Work out the finished part from the listing and answer in its coordinate system (mm). A direction names the side the tool comes from. Coordinates: 2 decimals unless noted, no trailing zeros. Loops run counter-clockwise (first coordinate to the right, second up) from the corner with the lowest first, then second, coordinate; pieces in that order, holes last. Notation, with made-up numbers: (-4, 14) -> (33, 14) arc R16 cw to (33, 37) -> close; hole circle Ø3 at (17, 70.25). An arc over 180 degrees is marked (long way). Use a Markdown table: item, result.
from build123d import *

# Parameters (mm, degrees)
SKETCH1_R                    = 9.45
BOSS_EXTRUDE1_DEPTH          = 7
SKETCH2_R                    = 8.95
BOSS_EXTRUDE2_DEPTH          = 2
SKETCH3_R                    = 9.45
BOSS_EXTRUDE3_DEPTH          = 7
SKETCH4_R                    = 4
CUT_EXTRUDE1_DEPTH           = 21.847182064
M2_5X0_45_TAPPED_HOLE1_D     = 2.1
M2_5X0_45_TAPPED_HOLE1_DEPTH = 7
M2_5X0_45_TAPPED_HOLE1_TIP   = 0.63090365
M2_5X0_45_TAPPED_HOLE2_D     = 2.1
M2_5X0_45_TAPPED_HOLE2_DEPTH = 7
M2_5X0_45_TAPPED_HOLE2_TIP   = 0.63090365


with BuildPart() as part:
    # Sketch1 → Boss-Extrude1 (new body)
    with BuildSketch(Plane.XY):
        Circle(SKETCH1_R)
    extrude(amount=BOSS_EXTRUDE1_DEPTH)

    # Sketch2 → Boss-Extrude2 (add)
    with BuildSketch(Plane.XY.offset(7)):
        Circle(SKETCH2_R)
    extrude(amount=BOSS_EXTRUDE2_DEPTH)

    # Sketch3 → Boss-Extrude3 (add)
    with BuildSketch(Plane.XY.offset(9)):
        Circle(SKETCH3_R)
    extrude(amount=BOSS_EXTRUDE3_DEPTH)

    # Sketch4 → Cut-Extrude1 (cut, through all)
    with BuildSketch(Plane.XY.offset(16)):
        Circle(SKETCH4_R)
    extrude(amount=-CUT_EXTRUDE1_DEPTH, mode=Mode.SUBTRACT)

    # M2.5x0.45 Tapped Hole1
    with Locations(Plane.XY.offset(16)):
        with Locations((0, -7), (0, 7)):
            Hole(M2_5X0_45_TAPPED_HOLE1_D / 2, depth=M2_5X0_45_TAPPED_HOLE1_DEPTH)
            with Locations((0, 0, -(M2_5X0_45_TAPPED_HOLE1_DEPTH + M2_5X0_45_TAPPED_HOLE1_TIP / 2))):  # 118° drill point
                Cone(0, M2_5X0_45_TAPPED_HOLE1_D / 2, M2_5X0_45_TAPPED_HOLE1_TIP, mode=Mode.SUBTRACT)

    # M2.5x0.45 Tapped Hole2
    with Locations(Plane(origin=(0, 0, 0), x_dir=(-1, 0, 0), z_dir=(0, 0, -1))):
        with Locations((0, 7), (0, -7)):
            Hole(M2_5X0_45_TAPPED_HOLE2_D / 2, depth=M2_5X0_45_TAPPED_HOLE2_DEPTH)
            with Locations((0, 0, -(M2_5X0_45_TAPPED_HOLE2_DEPTH + M2_5X0_45_TAPPED_HOLE2_TIP / 2))):  # 118° drill point
                Cone(0, M2_5X0_45_TAPPED_HOLE2_D / 2, M2_5X0_45_TAPPED_HOLE2_TIP, mode=Mode.SUBTRACT)


solid = part.part
Q1. Section B-B on y = 0 is taken. Determine the outline of the cut face in (x, z), and give its area (3 significant figures).
Solved:
| item | result |
|---|---|
| outline | (-9.45, 0) -> (-4, 0) -> (-4, 16) -> (-9.45, 16) -> (-9.45, 9) -> (-8.95, 9) -> (-8.95, 7) -> (-9.45, 7) -> close; (4, 0) -> (9.45, 0) -> (9.45, 7) -> (8.95, 7) -> (8.95, 9) -> (9.45, 9) -> (9.45, 16) -> (4, 16) -> close |
| area | 172 mm² |
Q2. Given pin 1 Ø1.3 at (x, y) = (0, 7) entering from -Z; pin 2 Ø1.9 at (x, y) = (0, -7) entering from +Z; pin 3 Ø6 at (x, z) = (-4, 13) entering from -Y, each flat-ended and moving along its own axis, determine where each tip first touches the part or whether it passes through.
Solved:
| item | result |
|---|---|
| pin 1 | z = 7.24 |
| pin 2 | z = 8.94 |
| pin 3 | y = -9.4 |
Q3. Section C-C on z = 10.5 is taken. Determine the outline of the cut face in (x, y).
Solved:
| item | result |
|---|---|
| outline | circle Ø18.9 at (0, 0); hole circle Ø8 at (0, 0); hole circle Ø2.1 at (0, -7); hole circle Ø2.1 at (0, 7) |
Q4. Determine the mould class of faces 1 (the cylindrical face through (9.014, 2.839, 12.451)), 2 (the flat face through (4, -2, 16)), 3 (the cylindrical face through (-0.14, -5.96, 3.55)) for opening direction Y: pulls with the +Y half, pulls with the -Y half, needs draft (parallel to the pull), parting line crosses it, or undercut.
Solved:
| item | result |
|---|---|
| face 1 | parting line crosses it |
| face 2 | needs draft |
| face 3 | undercut |
Q5. Section A-A on x = 3.25 is taken. Determine the outline of the cut face in (y, z).
Solved:
| item | result |
|---|---|
| outline | (-8.87, 0) -> (-2.33, 0) -> (-2.33, 16) -> (-8.87, 16) -> (-8.87, 9) -> (-8.34, 9) -> (-8.34, 7) -> (-8.87, 7) -> close; (2.33, 0) -> (8.87, 0) -> (8.87, 7) -> (8.34, 7) -> (8.34, 9) -> (8.87, 9) -> (8.87, 16) -> (2.33, 16) -> close |
Q6. Section D-D on x = -8 is taken. Determine the outline of the cut face in (y, z), and give its area (3 significant figures).
Solved:
| item | result |
|---|---|
| outline | (-5.03, 0) -> (5.03, 0) -> (5.03, 7) -> (4.01, 7) -> (4.01, 9) -> (5.03, 9) -> (5.03, 16) -> (-5.03, 16) -> (-5.03, 9) -> (-4.01, 9) -> (-4.01, 7) -> (-5.03, 7) -> close |
| area | 157 mm² |
Q7. For faces 4 (the cylindrical face through (-1.05, 7.05, 3.55)), 5 (the flat face through (4, -2, 0)), 6 (the flat face through (-6, -7, 9)), 7 (the cylindrical face through (0.14, -5.96, 12.45)), determine the directions among +Z, -Z, +X, -X, +Y, -Y from which every point of the face is accessible in a straight line to the end or side of a thin tool.
Solved:
| item | result |
|---|---|
| face 4 | -Z |
| face 5 | -Z, +X, -X, +Y, -Y |
| face 6 | none |
| face 7 | +Z |
Q8. Consider line 1 (Y direction, x = 0, z = 5.75); line 2 (Y direction, x = 0.5, z = 15.75); line 3 (Z direction, x = -5.25, y = -7.5). Determine where each line is inside the solid, lowest interval first. Write a range as [from, to].
Solved:
| item | result |
|---|---|
| line 1 | [-9.45, -8.05], [-5.95, -4], [4, 5.95], [8.05, 9.45] |
| line 2 | [-9.44, -7.92], [-6.08, -3.97], [3.97, 6.08], [7.92, 9.44] |
| line 3 | [0, 7], [9, 16] |
